The listing builds one solid part. Answer for the finished solid, in the listing's coordinates (mm). A direction names the side the tool comes from. Round coordinates to 2 decimals unless told otherwise and drop trailing zeros.
Item 1: Each of these flat-tipped pins is pushed along its axis until it touches: pin 1 (3.5 mm diameter, centred on x = 18.75, y = -16.75, fed in from -Z); pin 2 (1.2 mm diameter, centred on y = -18.5, z = 6.5, fed in from -X); pin 3 (3 mm diameter, centred on x = -18.75, y = 16.75, fed in from +Z). Where does it stop, or does it pass through?
Item 2: For a pull along Y with two mould halves and no side action, classify faces 6 (the face through (-22, 15, 4)), 7 (the face through (-18.475, -0.192, 3.812)), 8 (the face through (19.36, -19.42, 0.49)) as +Y half, -Y half, draft (parallel to the pull), parting line (faces both ways), or undercut.
Item 3: A tool of negligible diameter and unlimited length cuts with its end or side. For faces 1 (the face through (13.16, 15.69, 6.9)), 2 (the face through (14.02, -20, 8)), 3 (the face through (-0.3, -11.3, 6)), 4 (the face through (14.02, 20, 8)), 5 (the face through (16, 18, 9.25)), from which of +Z, -Z, +X, -X, +Y, -Y can it reach the whole face along a straight path? Write none if from no direction.
Item 4: Find section C-C on z = 7.5. Give the number of separate pieces and of enclosed holes in the cut face, then the cut area to 3 significant figures.
Item 5: Find the intervals of material crossed by probe 1 along X at (y, z) = (0, 2.5); probe 2 along Y at (x, z) = (18.75, 6.25); probe 3 along Y at (x, z) = (-18.75, 5.75), in increasing order.
```python
from build123d import *

# Parameters (mm, degrees)
CROQUIS1_W              = 44
CROQUIS1_H              = 44
CROQUIS1_R              = 12.1
SALIENTE_EXTRUIR1_DEPTH = 6
CHAFL_N2_SIZE           = 4.5
CROQUIS2_R              = 1.35
CORTAR_EXTRUIR1_DEPTH   = 32.685959036
CROQUIS3_R              = 21.308128052
CORTAR_EXTRUIR2_DEPTH   = 32.685959036
CHAFL_N4_SIZE           = 1
SALIENTE_EXTRUIR2_START = 3.25
CROQUIS4_R              = 1.35
SALIENTE_EXTRUIR2_DEPTH = 3.25
CHAFL_N5_SIZE           = 3
CHAFL_N3_SIZE           = 0.75
REDONDEO1_R             = 3
CROQUIS5_R              = 15.396724601
CROQUIS5_R_2            = 11
SALIENTE_EXTRUIR4_DEPTH = 1
CHAFL_N6_SIZE           = 1.5
CHAFL_N7_SIZE           = 1


# Some blends are built 0.0001 mm under size
with BuildPart() as part:
    # Croquis1 → Saliente-Extruir1 (new body)
    with BuildSketch(Plane.XY):
        Rectangle(CROQUIS1_W, CROQUIS1_H)
        Circle(CROQUIS1_R, mode=Mode.SUBTRACT)
    extrude(amount=SALIENTE_EXTRUIR1_DEPTH)

    # Chaflán2
    chafl_n2_edges = [part.edges().sort_by_distance(p)[0] for p in [
        (-22, 22, 3),
        (22, 22, 3),
        (22, -22, 3),
        (-22, -22, 3),
    ]]
    chamfer(chafl_n2_edges, length=CHAFL_N2_SIZE)

    # Croquis2 → Cortar-Extruir1 (cut, through all)
    with BuildSketch(Plane.XY.offset(6)):
        with Locations((-18.75, -16.75)):
            Circle(CROQUIS2_R)
        with Locations((18.75, -16.75)):
            Circle(CROQUIS2_R)
        with Locations((18.75, 16.75)):
            Circle(CROQUIS2_R)
        with Locations((-18.75, 16.75)):
            Circle(CROQUIS2_R)
    extrude(amount=-CORTAR_EXTRUIR1_DEPTH, mode=Mode.SUBTRACT)

    # Croquis3 → Cortar-Extruir2 (cut, through all)
    with BuildSketch(Plane.XY.offset(6)):
        with Locations((40.594273769, 0)):
            Circle(CROQUIS3_R)
        with Locations((-40.594273769, 0)):
            Circle(CROQUIS3_R)
        with BuildLine():
            Line((14.527768994, 48.750256971), (14.527768994, 30.973585325))
            ThreePointArc((14.527768994, 30.973585325), (0, 16.445816331), (-14.527768994, 30.973585325))
            Line((-14.527768994, 30.973585325), (-14.527768994, 48.750256971))
            ThreePointArc((-14.527768994, 48.750256971), (0, 63.278025965), (14.527768994, 48.750256971))
        make_face()
        with BuildLine():
            Line((14.527768994, -48.750256971), (14.527768994, -30.973585325))
            ThreePointArc((14.527768994, -30.973585325), (0, -16.445816331), (-14.527768994, -30.973585325))
            Line((-14.527768994, -30.973585325), (-14.527768994, -48.750256971))
            ThreePointArc((-14.527768994, -48.750256971), (0, -63.278025965), (14.527768994, -48.750256971))
        make_face()
    extrude(amount=-CORTAR_EXTRUIR2_DEPTH, mode=Mode.SUBTRACT)

    # Chaflán4
    chafl_n4_edges = [part.edges().sort_by_distance(p)[0] for p in [
        (-22, 13.953107343, 0),
        (14.462504669, 22, 0),
        (22, -13.953107343, 0),
        (-14.462504669, -22, 0),
        (19.75, -19.75, 0),
        (-19.75, -19.75, 0),
        (19.75, 19.75, 0),
        (-19.75, 19.75, 0),
        (-14.462504669, 22, 0),
        (22, 13.953107343, 0),
        (14.462504669, -22, 0),
        (-22, -13.953107343, 0),
        (19.286145717, 0, 0),
        (0, -16.445816331, 0),
        (0, 16.445816331, 0),
        (-19.286145717, 0, 0),
    ]]
    chamfer(chafl_n4_edges, length=CHAFL_N4_SIZE)

    # Croquis4 → Saliente-Extruir2 (add)
    # profile 1 of 4: a face of its own
    with BuildSketch(Plane.XY.offset(6).offset(SALIENTE_EXTRUIR2_START)):
        Polygon((-22, -17.5), (-17.5, -22), (-14.019564426, -22), (-14.019564426, -13.289292173), (-22, -13.289292173), align=None)
        with Locations((-18.75, -16.75)):
            Circle(CROQUIS4_R, mode=Mode.SUBTRACT)
    # profile 2 of 4: a face of its own
    with BuildSketch(Plane.XY.offset(6).offset(SALIENTE_EXTRUIR2_START)):
        Polygon((22, -13.289292173), (22, -17.5), (17.5, -22), (14.019564426, -22), (14.019564426, -13.289292173), align=None)
        with Locations((18.75, -16.75)):
            Circle(CROQUIS4_R, mode=Mode.SUBTRACT)
    # profile 3 of 4: a face of its own
    with BuildSketch(Plane.XY.offset(6).offset(SALIENTE_EXTRUIR2_START)):
        Polygon((22, 17.5), (17.5, 22), (14.019564426, 22), (14.019564426, 13.289292173), (22, 13.289292173), align=None)
        with Locations((18.75, 16.75)):
            Circle(CROQUIS4_R, mode=Mode.SUBTRACT)
    # profile 4 of 4: a face of its own
    with BuildSketch(Plane.XY.offset(6).offset(SALIENTE_EXTRUIR2_START)):
        Polygon((-22, 13.289292173), (-22, 17.5), (-17.5, 22), (-14.019564426, 22), (-14.019564426, 13.289292173), align=None)
        with Locations((-18.75, 16.75)):
            Circle(CROQUIS4_R, mode=Mode.SUBTRACT)
    extrude(amount=-SALIENTE_EXTRUIR2_DEPTH)

    # Chaflán5
    chafl_n5_edges = [part.edges().sort_by_distance(p)[0] for p in [
        (-19.286145717, 0, 6),
        (19.286145717, 0, 6),
        (0, -16.445816331, 6),
        (0, 16.445816331, 6),
    ]]
    chamfer(chafl_n5_edges, length=CHAFL_N5_SIZE)

    # Chaflán3
    # the kernel refuses this chamfer: 0.75 mm, written as the material it takes off along each edge
    with BuildSketch(Plane(origin=(-18.75, -16.75, 9.25), x_dir=(1, 0, 0), z_dir=(0, -1, 0))) as chafl_n3_piece_1:
        Polygon((1.35, -CHAFL_N3_SIZE), (1.35 + CHAFL_N3_SIZE, 0), (1.35, 0), align=None)
    revolve(axis=Axis((-18.75, -16.75, 9.25), (0, 0, 1)), mode=Mode.SUBTRACT)
    with BuildSketch(Plane(origin=(18.75, -16.75, 9.25), x_dir=(1, 0, 0), z_dir=(0, -1, 0))) as chafl_n3_piece_2:
        Polygon((1.35, -CHAFL_N3_SIZE), (1.35 + CHAFL_N3_SIZE, 0), (1.35, 0), align=None)
    revolve(axis=Axis((18.75, -16.75, 9.25), (0, 0, 1)), mode=Mode.SUBTRACT)
    with BuildSketch(Plane(origin=(18.75, 16.75, 9.25), x_dir=(1, 0, 0), z_dir=(0, -1, 0))) as chafl_n3_piece_3:
        Polygon((1.35 + CHAFL_N3_SIZE, 0), (1.35, -CHAFL_N3_SIZE), (1.35, 0), align=None)
    revolve(axis=Axis((18.75, 16.75, 9.25), (0, 0, 1)), mode=Mode.SUBTRACT)
    with BuildSketch(Plane(origin=(-18.75, 16.75, 9.25), x_dir=(1, 0, 0), z_dir=(0, -1, 0))) as chafl_n3_piece_4:
        Polygon((1.35 + CHAFL_N3_SIZE, 0), (1.35, -CHAFL_N3_SIZE), (1.35, 0), align=None)
    revolve(axis=Axis((-18.75, 16.75, 9.25), (0, 0, 1)), mode=Mode.SUBTRACT)
    with BuildSketch(Plane(origin=(-18.75, 16.75, 0), x_dir=(1, 0, 0), z_dir=(0, -1, 0))) as chafl_n3_piece_5:
        Polygon((1.35 + CHAFL_N3_SIZE, 0), (1.35, CHAFL_N3_SIZE), (1.35, 0), align=None)
    revolve(axis=Axis((-18.75, 16.75, 0), (0, 0, 1)), mode=Mode.SUBTRACT)
    with BuildSketch(Plane(origin=(18.75, 16.75, 0), x_dir=(1, 0, 0), z_dir=(0, -1, 0))) as chafl_n3_piece_6:
        Polygon((1.35 + CHAFL_N3_SIZE, 0), (1.35, CHAFL_N3_SIZE), (1.35, 0), align=None)
    revolve(axis=Axis((18.75, 16.75, 0), (0, 0, 1)), mode=Mode.SUBTRACT)
    with BuildSketch(Plane(origin=(18.75, -16.75, 0), x_dir=(1, 0, 0), z_dir=(0, -1, 0))) as chafl_n3_piece_7:
        Polygon((1.35 + CHAFL_N3_SIZE, 0), (1.35, CHAFL_N3_SIZE), (1.35, 0), align=None)
    revolve(axis=Axis((18.75, -16.75, 0), (0, 0, 1)), mode=Mode.SUBTRACT)
    with BuildSketch(Plane(origin=(-18.75, -16.75, 0), x_dir=(1, 0, 0), z_dir=(0, -1, 0))) as chafl_n3_piece_8:
        Polygon((1.35 + CHAFL_N3_SIZE, 0), (1.35, CHAFL_N3_SIZE), (1.35, 0), align=None)
    revolve(axis=Axis((-18.75, -16.75, 0), (0, 0, 1)), mode=Mode.SUBTRACT)

    # Redondeo1
    redondeo1_edges = [part.edges().sort_by_distance(p)[0] for p in [
        (14.019564426, -16.871341335, 6),
        (-14.019564426, 16.871341335, 6),
        (-14.019564426, -16.871341335, 6),
        (14.019564426, 16.871341335, 6),
    ]]
    fillet(redondeo1_edges, radius=REDONDEO1_R)

    # Croquis5 → Saliente-Extruir4 (add)
    with BuildSketch(Plane(origin=(0, 0, 6), x_dir=(-1, 0, 0), z_dir=(0, 0, -1))):
        Circle(CROQUIS5_R)
        Circle(CROQUIS5_R_2, mode=Mode.SUBTRACT)
    extrude(amount=SALIENTE_EXTRUIR4_DEPTH)

    # Chaflán6
    chafl_n6_edges = [part.edges().sort_by_distance(p)[0] for p in [
        (-12.1, 0, 0),
    ]]
    chamfer(chafl_n6_edges, length=CHAFL_N6_SIZE)

    # Chaflán7
    chafl_n7_edges = [part.edges().sort_by_distance(p)[0] for p in [
        (11, 0, 5),
    ]]
    chamfer(chafl_n7_edges, length=CHAFL_N7_SIZE - 0.0001)  # a hair under: the kernel refuses the full size


solid = part.part
```
Check values:
1. pin 1: stops at z = 0.35
1. pin 2: stops at x = -21.6
1. pin 3: stops at z = 8.65
2. face 6: draft
2. face 7: undercut
2. face 8: -Y half
3. face 1: +Z, +Y, -Y
3. face 2: +Z, -Y
3. face 3: +Z
3. face 4: +Z, +Y
3. face 5: +Z, +X, -X, +Y, -Y
4. separate pieces: 4
4. enclosed holes: 4
4. area: 222 mm2
5. probe 1: x = -19.29 to -12.1, 12.1 to 19.29
5. probe 2: y = -20.75 to -18.1, -15.4 to -13.29, 13.29 to 15.4, 18.1 to 20.75
5. probe 3: y = -20.75 to -18.1, -15.4 to -10.08, 10.08 to 15.4, 18.1 to 20.75
